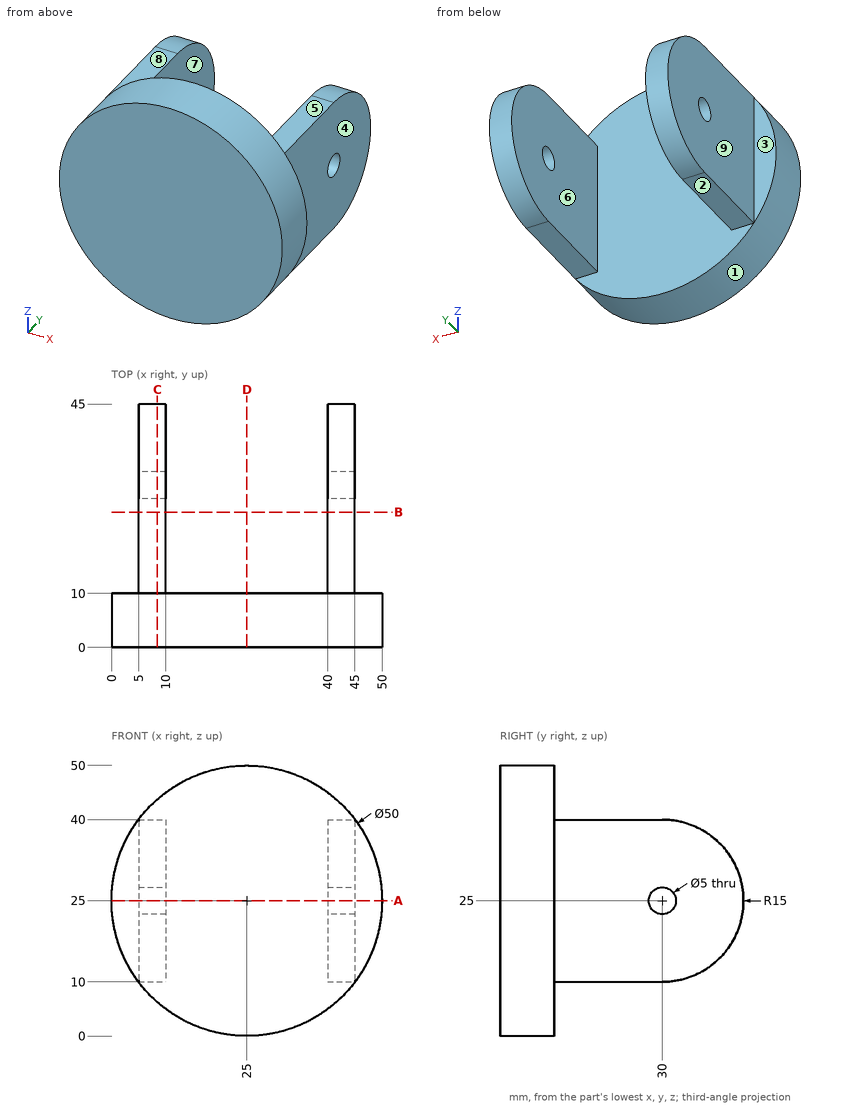
The figure shows three views and two pictorial views of one solid part (mm, origin at its lowest corner). Answer the questions. A direction names the side the tool comes from. Round coordinates to 2 decimals unless told otherwise and drop trailing zeros. Write each loop counter-clockwise with the first axis right and the second up, starting at its lowest first coordinate (ties: lowest second). Pieces come first, ordered by that corner, then holes. Notation, with made-up numbers: (8.25, 55) -> (63.25, 55) arc R22 cw to (63.25, 80) -> close; hole circle Ø6 at (42, -3). An arc over 180 degrees is marked (long way). Answer as a JSON object with one key per item and string values. Group by question number.
Q1. Section A-A (z = 25) is taken. Write down the section's boundary in (x, y), plus the area to 3 significant figures.
Q2. Determine the mould class of the marked faces 6, 7, 8 and 9 for opening direction X: pulls with the +X half, pulls with the -X half, needs draft (parallel to the pull), parting line crosses it, or undercut.
Q3. Section B-B (y = 25) is taken. Write down the section's boundary in (x, z).
Q4. Each of these flat-tipped pins is pushed along its axis until it touches: pin 1 Ø5.5 at (x, z) = (1.5, 32) entering from +Y; pin 2 Ø1 at (y, z) = (31, 40) entering from +X; pin 3 Ø2 at (x, z) = (33, 27.5) entering from -Y; pin 4 Ø5.5 at (x, y) = (41.5, 21.5) entering from -Z. Where does it stop, or does it pass through?
Q5. Section D-D (x = 25) is taken. Write down the section's boundary in (y, z).
Q6. Section C-C (x = 8.5) is taken. Write down the section's boundary in (y, z).
Q7. Straight lines are drawn through the part: line 1 along Y through (x, z) = (42, 25); line 2 along X through (y, z) = (41.5, 31); line 3 along Y through (x, z) = (27.5, 9). For each, find the intervals that lie inside material, in ascending order.
Q8. Which of the six approach directions +Z, -Z, +X, -X, +Y, -Y give full straight-line access (tool end or side, diameter ignored) to the marked faces 1, 2, 3, 4 and 5?
Check values:
{
 "1": {"outline": "(0, 0) -> (50, 0) -> (50, 10) -> (45, 10) -> (45, 27.5) -> (40, 27.5) -> (40, 10) -> (10, 10) -> (10, 27.5) -> (5, 27.5) -> (5, 10) -> (0, 10) -> close; (5, 32.5) -> (10, 32.5) -> (10, 45) -> (5, 45) -> close; (40, 32.5) -> (45, 32.5) -> (45, 45) -> (40, 45) -> close", "area": "800 mm^2"},
 "2": {"face 6": "undercut", "face 7": "undercut", "face 8": "needs draft", "face 9": "pulls with the -X half"},
 "3": {"outline": "(5, 10) -> (10, 10) -> (10, 40) -> (5, 40) -> close; (40, 10) -> (45, 10) -> (45, 40) -> (40, 40) -> close"},
 "4": {"pin 1": "y = 10", "pin 2": "x = 45", "pin 3": "y = 0", "pin 4": "z = 10"},
 "5": {"outline": "(0, 0) -> (10, 0) -> (10, 50) -> (0, 50) -> close"},
 "6": {"outline": "(0, 6.22) -> (10, 6.22) -> (10, 10) -> (30, 10) arc R15 ccw to (30, 40) -> (10, 40) -> (10, 43.78) -> (0, 43.78) -> close; hole circle Ø5 at (30, 25)"},
 "7": {"line 1": "0 to 27.5, 32.5 to 45", "line 2": "5 to 10, 40 to 45", "line 3": "0 to 10"},
 "8": {"face 1": "+Y, -Y", "face 2": "-Z, +X, -X, +Y", "face 3": "+Z, -Z, -X, +Y", "face 4": "+Z, -Z, +X, +Y", "face 5": "+Z, +X, -X, +Y"}
}
